```python
from build123d import *

# Parameters (mm, degrees)
SKIZZE2_R                       = 1.825
AUFSATZ_LINEAR_AUSTRAGEN1_DEPTH = 10
SCHNITT_LINEAR_AUSTRAGEN1_DEPTH = 11


with BuildPart() as part:
    # Skizze2 → Aufsatz-Linear austragen1 (new body)
    with BuildSketch(Plane(origin=(0, 0, 0), x_dir=(1, 0, 0), z_dir=(0, 1, 0))):
        with BuildLine():
            Line((0, 3.5), (-26.846787517, 3.5))
            Line((-26.846787517, 3.5), (-40.270181276, 26.75))
            ThreePointArc((-40.270181276, 26.75), (-45.051270189, 28.031088913), (-46.332359102, 23.25))
            Line((-46.332359102, 23.25), (-30.888239402, -3.5))
            Line((-30.888239402, -3.5), (0, -3.5))
            ThreePointArc((0, -3.5), (3.5, 0), (0, 3.5))
        make_face()
        with Locations((-43.301270189, 25)):
            Circle(SKIZZE2_R, mode=Mode.SUBTRACT)
        Circle(SKIZZE2_R, mode=Mode.SUBTRACT)
    extrude(amount=AUFSATZ_LINEAR_AUSTRAGEN1_DEPTH)

    # Skizze4 → Schnitt-Linear austragen1 (cut, through all)
    with BuildSketch(Plane(origin=(0, 10, 0), x_dir=(1, 0, 0), z_dir=(0, 1, 0))):
        with BuildLine():
            Line((-36.135462652, 16.588457268), (-27.135462652, 1))
            ThreePointArc((-27.135462652, 1), (-27.867513459, -1.732050808), (-30.599564267, -1))
            Line((-30.599564267, -1), (-39.599564267, 14.588457268))
            ThreePointArc((-39.599564267, 14.588457268), (-38.867513459, 17.320508076), (-36.135462652, 16.588457268))
        make_face()
    extrude(amount=-SCHNITT_LINEAR_AUSTRAGEN1_DEPTH, mode=Mode.SUBTRACT)


solid = part.part
```
CAD build for the part. Positions are in the model's coordinates, mm. A direction names the side the tool comes from. Coordinates: 2 decimals unless noted, no trailing zeros. Write each loop counter-clockwise with the first axis right and the second up, starting at its lowest first coordinate (ties: lowest second). Pieces come first, ordered by that corner, then holes.
(1) Drill centre lines: probe 1 along Z at (x, y) = (0, 5.5) (3 decimals); probe 2 along Z at (x, y) = (-8, 5.25); probe 3 along X at (y, z) = (7.5, -13). Where is each one in solid material? Low to high.
(2) Cut at C-C, the plane x = -5.5. List the corners of the cut face in (y, z), and give its area (3 significant figures).
(3) 3-axis set-ups, long thin cutter, end or side, ignore diameter. For faces 5 (the face through (-35.04, 5.07, -6.69)), 6 (the face through (-24, 0, -3)), 7 (the face through (-13, 5, -3.5)): which of +Z, -Z, +X, -X, +Y, -Y reach the whole face in a straight line?
(4) Cut at D-D, the plane z = -11.5. List the corners of the cut face in (x, y).
(5) Cut at A-A, the plane y = 1.5. List the corners of the cut face in (x, z) (3 decimals).
(6) Two-plate mould, pull along X, no slides. Class faces 1 (the face through (-16, 5, 3.5)), 2 (the face through (-33.465, 4.93, -14.962)), 3 (the face through (-41.615, 4.93, -24.301)), 4 (the face through (-31.698, 5.07, -8.903)): +X half, -X half, draft (parallel to the pull), parting line (faces both ways), or undercut.
(7) Flat gauge pins, fed straight in: pin 1 (3 mm diameter, centred on x = -11, y = 2, fed in from -Z); pin 2 (10 mm diameter, centred on x = -36, z = -19, fed in from -Y); pin 3 (6 mm diameter, centred on x = -38, y = 7.5, fed in from +Z); pin 4 (2 mm diameter, centred on y = 5.5, z = -14, fed in from +X). Where does each tip first touch, or does it go through?
(8) Cut at B-B, the plane z = -3. List the corners of the cut face in (x, y), and give its area (3 significant figures).
Geometry says:
1. probe 1: z = -3.5 to -1.825, 1.825 to 3.5
1. probe 2: z = -3.5 to 3.5
1. probe 3: x = -40.41 to -38.68, -34.06 to -32.33
2. outline: (0, -3.5) - (10, -3.5) - (10, 3.5) - (0, 3.5) - close
2. area: 70.0 mm2
3. face 5: +Y, -Y
3. face 6: +Z, -Z, +X, -X, -Y
3. face 7: -Z, +X, +Y, -Y
4. outline: (-39.55, 0) - (-37.82, 0) - (-37.82, 10) - (-39.55, 10) - close; (-33.2, 0) - (-31.47, 0) - (-31.47, 10) - (-33.2, 10) - close
5. outline: (-46.332, -23.25) arc R3.5 ccw to (-40.27, -26.75) - (-26.847, -3.5) - (0, -3.5) arc R3.5 ccw to (0, 3.5) - (-30.888, 3.5) - close; hole circle Ø3.65 at (-43.301, -25); hole (-39.6, -14.588) arc R2 ccw to (-36.135, -16.588) - (-27.135, -1) arc R2 ccw to (-30.6, 1) - close; hole circle Ø3.65 at (0, 0)
6. face 1: draft
6. face 2: +X half
6. face 3: undercut
6. face 4: undercut
7. pin 1: stops at z = -3.5
7. pin 2: stops at y = 0
7. pin 3: stops at z = -3.62
7. pin 4: stops at x = -32.33
8. outline: (-34.64, 0) - (-32.91, 0) - (-32.91, 10) - (-34.64, 10) - close; (-28.29, 0) - (1.8, 0) - (1.8, 10) - (-28.29, 10) - close
8. area: 318 mm2
